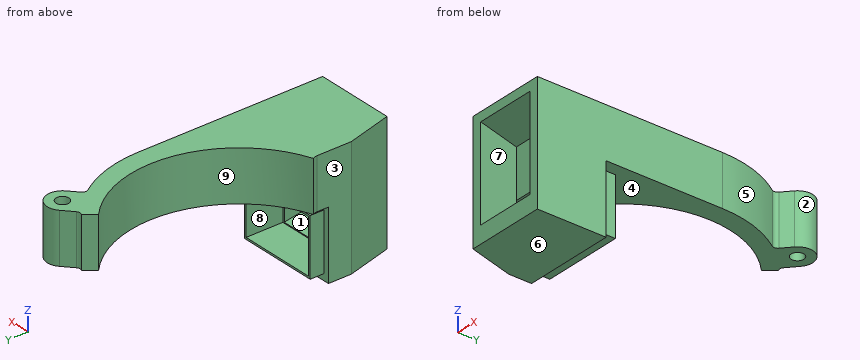
```python
from build123d import *

# Parameters (mm, degrees)
SKETCH1_R               = 1.4
BOSS_EXTRUDE1_DEPTH     = 11
SKETCH2_W               = 18.000000053
SKETCH2_H               = 12.9
SKETCH2_W_2             = 16.800000053
SKETCH2_H_2             = 11.7
BOSS_EXTRUDE2_DEPTH     = 3
SKETCH2_3_W             = 20
SKETCH2_3_H             = 11
SKETCH2_3_H_2           = 15
SKETCH2_3_W_2           = 18.000000053
SKETCH2_3_H_3           = 12.9
SKETCH2_3_W_3           = 16.800000053
SKETCH2_3_H_4           = 11.7
BOSS_EXTRUDE3_DEPTH     = 5
BOSS_EXTRUDE4_DEPTH     = 2
BOSS_EXTRUDE6_START     = -2
BOSS_EXTRUDE6_DEPTH     = 22
SKETCH4_3_W             = 2
SKETCH4_3_H             = 40
BOSS_EXTRUDE6_2_DEPTH   = 22
BOSS_EXTRUDE7_START     = -24
SKETCH4_4_W             = 2
SKETCH4_4_H             = 40
BOSS_EXTRUDE7_DEPTH     = 2
BOSS_EXTRUDE8_REACH     = 20.326
SKETCH2_5_W             = 18.000000053
SKETCH2_5_H             = 12.9
SKETCH2_5_W_2           = 17.600000053
SKETCH2_5_H_2           = 12.5
CUT_EXTRUDE_THIN6_DEPTH = 10
SKETCH11_W              = 50.134644107
SKETCH11_H              = 30
CUT_EXTRUDE6_DEPTH      = 27


with BuildPart() as part:
    # Sketch1 → Boss-Extrude1 (new body)
    with BuildSketch(Plane.XY):
        with BuildLine():
            Line((23.20688118, 15.778885673), (25.185252728, 17.527214018))
            ThreePointArc((25.185252728, 17.527214018), (25.472785982, 22.185252728), (20.814747272, 22.472785982))
            Line((20.814747272, 22.472785982), (18.598905377, 20.514600122))
            ThreePointArc((18.598905377, 20.514600122), (17.974550182, 20.264645495), (17.333078903, 20.466663618))
            Line((17.333078903, 20.466663618), (15.586200014, 18.159406728))
            ThreePointArc((15.586200014, 18.159406728), (22.681435087, -4.226534244), (7.174093823, -21.861586862))
            ThreePointArc((7.174093823, -21.861586862), (7.416792587, -22.384967182), (7.5, -22.955849111))
            Line((7.5, -22.955849111), (7.5, -25.4))
            Line((7.5, -25.4), (27.5, -25.4))
            Line((27.5, -25.4), (27.5, 0))
            ThreePointArc((27.5, 0), (26.362874376, 7.569397218), (23.04284729, 14.466226133))
            ThreePointArc((23.04284729, 14.466226133), (22.876796583, 15.153555184), (23.20688118, 15.778885673))
        make_face()
        with Locations((23, 20)):
            Circle(SKETCH1_R, mode=Mode.SUBTRACT)
    extrude(amount=BOSS_EXTRUDE1_DEPTH)



with BuildPart() as body_2:
    # Sketch2 → Boss-Extrude2 (new body)
    with BuildSketch(Plane.XZ.offset(25.4)):
        with Locations((17.500000027, -7.35)):
            Rectangle(SKETCH2_W, SKETCH2_H)
        with Locations((17.500000027, -7.35)):
            Rectangle(SKETCH2_W_2, SKETCH2_H_2, mode=Mode.SUBTRACT)
    extrude(amount=-BOSS_EXTRUDE2_DEPTH)


with BuildPart() as part_1:
    add(part.part)

    add(body_2.part)  # Boss-Extrude3 merges body 2
    # Sketch2<3> → Boss-Extrude3 (add)
    with BuildSketch(Plane.XZ.offset(25.4)):
        with Locations((17.5, 5.5)):
            Rectangle(SKETCH2_3_W, SKETCH2_3_H)
        with Locations((17.5, -7.5)):
            Rectangle(SKETCH2_3_W, SKETCH2_3_H_2)
        with Locations((17.500000027, -7.35)):
            Rectangle(SKETCH2_3_W_2, SKETCH2_3_H_3, mode=Mode.SUBTRACT)
        with Locations((17.500000027, -7.35)):
            Rectangle(SKETCH2_3_W_2, SKETCH2_3_H_3)
        with Locations((17.500000027, -7.35)):
            Rectangle(SKETCH2_3_W_3, SKETCH2_3_H_4, mode=Mode.SUBTRACT)
    extrude(amount=BOSS_EXTRUDE3_DEPTH)

    # Sketch4 → Boss-Extrude4 (add)
    with BuildSketch(Plane(origin=(0, 0, -15), x_dir=(-1, 0, 0), z_dir=(0, 0, -1))):
        Polygon((-18.42672165, -70.4), (-7.5, -30.4), (-27.5, -30.4), (-27.5, -70.4), align=None)
    extrude(amount=-BOSS_EXTRUDE4_DEPTH)



with BuildPart() as body_2_2:
    # Sketch4<3> → Boss-Extrude6 (new body)
    with BuildSketch(Plane(origin=(0, 0, -15), x_dir=(-1, 0, 0), z_dir=(0, 0, -1)).offset(BOSS_EXTRUDE6_START)):
        Polygon((-18.42672165, -70.4), (-7.5, -30.4), (-9.57327835, -30.4), (-20.5, -70.4), align=None)
    extrude(amount=-BOSS_EXTRUDE6_DEPTH)


with BuildPart() as body_3:
    # Sketch4<3> → Boss-Extrude6 2 (new body)
    with BuildSketch(Plane(origin=(0, 0, -15), x_dir=(-1, 0, 0), z_dir=(0, 0, -1)).offset(BOSS_EXTRUDE6_START)):
        with Locations((-26.5, -50.4)):
            Rectangle(SKETCH4_3_W, SKETCH4_3_H)
    extrude(amount=-BOSS_EXTRUDE6_2_DEPTH)


with BuildPart() as part_2:
    add(part_1.part)

    add(body_2_2.part)  # Boss-Extrude7 merges body 2 2

    add(body_3.part)  # Boss-Extrude7 merges body 3
    # Sketch4<4> → Boss-Extrude7 (add)
    with BuildSketch(Plane(origin=(0, 0, -15), x_dir=(-1, 0, 0), z_dir=(0, 0, -1)).offset(BOSS_EXTRUDE7_START)):
        Polygon((-20.5, -70.4), (-9.57327835, -30.4), (-25.5, -30.4), (-25.5, -70.4), align=None)
        Polygon((-18.42672165, -70.4), (-7.5, -30.4), (-9.57327835, -30.4), (-20.5, -70.4), align=None)
        with Locations((-26.5, -50.4)):
            Rectangle(SKETCH4_4_W, SKETCH4_4_H)
    extrude(amount=-BOSS_EXTRUDE7_DEPTH)

    # Boss-Extrude8: up to this face of the body (flat: up to its plane)
    boss_extrude8_end = Plane(part_2.part.faces().sort_by_distance((15.036639175, -50.4, -2))[0])
    # Sketch8 → Boss-Extrude8 (add, up to the picked face)
    with BuildSketch(Plane.ZY.offset(-25.5), mode=Mode.PRIVATE) as boss_extrude8_sk1:
        Polygon((-13, -70.4), (-6, -70.4), (-13, -30.4), align=None)
    boss_extrude8_tool1 = split(extrude(boss_extrude8_sk1.sketch, amount=BOSS_EXTRUDE8_REACH, mode=Mode.PRIVATE), bisect_by=boss_extrude8_end, keep=Keep.BOTH, mode=Mode.PRIVATE)
    add(boss_extrude8_tool1.solids().sort_by_distance((25.5, -57.066667, -10.666667))[0])

    # Sketch2<5> → Cut-Extrude-Thin6 (cut)
    with BuildSketch(Plane.XZ.offset(25.4)):
        with Locations((17.500000027, -7.35)):
            Rectangle(SKETCH2_5_W, SKETCH2_5_H)
        with Locations((17.500000027, -7.35)):
            Rectangle(SKETCH2_5_W_2, SKETCH2_5_H_2, mode=Mode.SUBTRACT)
    extrude(amount=-CUT_EXTRUDE_THIN6_DEPTH, mode=Mode.SUBTRACT)

    # Sketch11 → Cut-Extrude6 (cut, through all)
    with BuildSketch(Plane(origin=(0, 0, -15), x_dir=(-1, 0, 0), z_dir=(0, 0, -1))):
        with Locations((-25.067322053, -55.4)):
            Rectangle(SKETCH11_W, SKETCH11_H)
    extrude(amount=-CUT_EXTRUDE6_DEPTH, mode=Mode.SUBTRACT)


solid = part_2.part
```
Source: CAD feature listing. Evaluate the final solid. Frame: model axes, mm. Face numbers are marked on the shaded views. A direction names the side the tool comes from. Give positions to 0.01 mm unless a question says otherwise; leave off trailing zeros. Order: outer loops, then holes, each group sorted by start corner. A loop starts at its lowest first (then second) coordinate and runs counter-clockwise, first axis right, second up. Notation, with made-up numbers: (55.25, -9.75) -> (110.25, -9.75) arc R27 cw to (110.25, 7.25) -> close; hole circle Ø6 at (58, -39). An arc over 180 degrees is marked (long way). Use a Markdown table: item, result.
Q1. Pull-direction query (Z, two-part tool) for the marked faces 6, 7, 8 and 9; classes: +Z half, -Z half, draft (parallel to the pull), parting line (faces both ways), or undercut.
A:
| item | result |
|---|---|
| face 6 | -Z half |
| face 7 | undercut |
| face 8 | undercut |
| face 9 | draft |
Q2. Section A-A (z = -5.5). Return the cut outline in (x, y).
A:
| item | result |
|---|---|
| outline | (7.5, -30.4) -> (10.23, -40.4) -> (12.3, -40.4) -> (9.57, -30.4) -> (9.1, -30.4) -> (9.1, -22.4) -> (8.7, -22.4) -> (8.7, -25.4) -> (7.5, -25.4) -> close; (25.5, -40.4) -> (27.5, -40.4) -> (27.5, -25.4) -> (26.3, -25.4) -> (26.3, -22.4) -> (25.9, -22.4) -> (25.9, -30.4) -> (25.5, -30.4) -> close |
Q3. Section C-C (y = -11). Return the cut outline in (x, z).
A:
| item | result |
|---|---|
| outline | (20.14, 0) -> (27.5, 0) -> (27.5, 11) -> (20.14, 11) -> close |
Q4. Access query for the marked faces 1, 2, 3, 4 and 5. Directions: +Z, -Z, +X, -X, +Y, -Y. A direction counts if a zero-diameter tool reaches every point of the face in a straight line with its end or side. Return the directions, or none.
A:
| item | result |
|---|---|
| face 1 | +Y |
| face 2 | +Z, -Z |
| face 3 | +Z, -Z, -X, -Y |
| face 4 | +X, -X, +Y |
| face 5 | +Z, -Z, +X |
Q5. Material intervals for line 1 (Z direction, x = 14.75, y = -23); line 2 (Y direction, x = 10.5, z = -14); line 3 (Z direction, x = 14, y = -29), sorted ascending. Write a range as [from, to].
A:
| item | result |
|---|---|
| line 1 | [-13.6, -13.2], [-1.5, -1.1], [0, 11] |
| line 2 | [-40.4, -25.4] |
| line 3 | [-15, -13.2], [-1.5, 11] |
Q6. First-contact query: P1, Ø4, axis at x = 16.5, z = 2, coming from the -Y side; P2, Ø4.5, axis at x = 16.5, z = -11, coming from the +Y side; P3, Ø0.9, axis at y = -24.5, z = -9.5, coming from the -X side. Flat tips, straight axial feed; report the tip coordinate or a pass-through.
A:
| item | result |
|---|---|
| P1 | y = -30.4 |
| P2 | y = -22.4 |
| P3 | x = 8.7 |
Q7. Section B-B (y = -1.5). Return the cut outline in (x, z).
A:
| item | result |
|---|---|
| outline | (23.09, 0) -> (27.5, 0) -> (27.5, 11) -> (23.09, 11) -> close |
